Model file for the job. Use its own axes, mm. A direction names the side the tool comes from. Give positions to 0.01 mm unless a question says otherwise; leave off trailing zeros. Order: outer loops, then holes, each group sorted by start corner. A loop starts at its lowest first (then second) coordinate and runs counter-clockwise, first axis right, second up. Notation, with made-up numbers: (-9.75, 21.25) - (39.25, 21.25) arc R29 cw to (39.25, 60.25) - close; hole circle Ø1 at (75, 74.5). An arc over 180 degrees is marked (long way). Use CSV: the item, a comma, the result in double quotes. Start each with the question number.
(1) Band-saw the part on B-B, the plane y = -2. Give the cut face in (x, z) (3 decimals), then the cut area to 3 significant figures.
(2) Drop flat-ended pins along their axis: pin 1 Ø2 at (x, z) = (0.5, 0.5) entering from +Y; pin 2 Ø2 at (y, z) = (-3.5, 2) entering from +X; pin 3 Ø1.2 at (x, z) = (-0.5, -0.5) entering from -Y; pin 4 Ø2.5 at (x, z) = (0, -7.5) entering from -Y. Give the stop position or say it passes through.
(3) Band-saw the part on A-A, the plane z = -7.5. Count the separate pieces of the cut face and the enclosed holes in it, then the cut area to 3 significant figures.
(4) Pull direction X, two halves, no side cores. Call faces 5 (the cylindrical face through (0.07, -5.51, -9)), 6 (the flat face through (1, 6, 2)), 7 (the conical face through (-1.88, 0.24, -5.95)), 8 (the cylindrical face through (0, 3, -6)): +X half, -X half, draft (parallel to the pull), parting line (faces both ways), or undercut.
(5) Probe L1, parallel to Y at x = 0, z = 5 (3 decimals); L2, parallel to X at y = 5.4, z = 0; L3, parallel to X at y = 5.7, z = 0. List the from-to ranges inside material, lowest first.
(6) Tool access for faces 1 (the flat face through (0, 1, 1.7)), 2 (the cylindrical face through (0.186, -0.587, 3.808)), 3 (the flat face through (5, -5, 5)), 4 (the flat face through (0, 5, 0)): list every direction of +Z, -Z, +X, -X, +Y, -Y with a clear straight run to the whole face (end or side of a thin tool).
from build123d import *

# Parameters (mm, degrees)
FLAT_GROVE_EXTRUDE_REACH   = 21.647
WIRE_HOLE_CUT_DEPTH        = 20.052558883
WIRE_HOLE_CUT_DEPTH_BACK   = 20.052558883
SKETCH5_R                  = 1.5
SKETCH6_R                  = 1.425
SET_SCREW_CUT_DEPTH        = 18.698870187
MAGNET_START               = -1
SKETCH8_R                  = 11
SKETCH8_R_2                = 3.05
MAGNET_HOLDER_TRIM_DEPTH   = 1
MAGNET_HOLDER_CHAMFER_SIZE = 1
AXLE_TOLERANCE_CUT_DEPTH   = 8


with BuildPart() as part:
    # Sketch1 → Spool Solid (revolve)
    with BuildSketch(Plane(origin=(0, 0, 0), x_dir=(0, 0, -1), z_dir=(1, 0, 0)), mode=Mode.PRIVATE) as spool_solid_sk:
        Polygon((-2.05, 6), (-11, 6), (-11, 5), (-6, 0), (-6, -5), (-11, -5), (-11, -6), (-2, -6), (-2, 2), (0, 4), (0, 5), (-2.05, 5), align=None)
    revolve(spool_solid_sk.sketch.rotate(Axis((0, 0, 0), (0, 1, 0)), 180), axis=Axis((0, 0, 0), (0, 1, 0)))

    # Flat Grove Extrude: up to this cone (the profile starts inside it)
    flat_grove_extrude_end = Plane(origin=(0, -6, 0), z_dir=(0, -1, 0)).offset(-9.999999) * Cone(1e-06, 42.147, 42.146999, align=(Align.CENTER, Align.CENTER, Align.MIN), mode=Mode.PRIVATE)
    # Sketch2 → Flat Grove Extrude (add, up to the surface)
    with BuildSketch(Plane.XZ.offset(6), mode=Mode.PRIVATE) as flat_grove_extrude_sk1:
        with BuildLine():
            Line((1.322875656, 1.5), (-1.322875656, 1.5))
            ThreePointArc((-1.322875656, 1.5), (0, 2), (1.322875656, 1.5))
        make_face()
    flat_grove_extrude_tool1 = extrude(flat_grove_extrude_sk1.sketch, amount=-FLAT_GROVE_EXTRUDE_REACH, mode=Mode.PRIVATE) & flat_grove_extrude_end
    add(flat_grove_extrude_tool1.solids().sort_by_distance((0, -6, 1.702311))[0])

    # Sketch5 → Wire Hole Cut (cut, two sides: drawn at the far end of the back side and taken through both)
    with BuildSketch(Plane(origin=(0, -5, 0), x_dir=(1, 0, 0), z_dir=(0, 1, 0)).offset(-WIRE_HOLE_CUT_DEPTH_BACK)):
        with Locations(Location((0, 7.5, 0), (0, 0, 270))):
            Circle(SKETCH5_R)
    extrude(amount=WIRE_HOLE_CUT_DEPTH + WIRE_HOLE_CUT_DEPTH_BACK, mode=Mode.SUBTRACT)

    # Sketch6 → Set Screw Cut (cut, through all)
    with BuildSketch(Plane(origin=(0, 0, 1.5), x_dir=(-1, 0, 0), z_dir=(0, 0, -1))):
        with Locations((0, -2)):
            Circle(SKETCH6_R)
    extrude(amount=-SET_SCREW_CUT_DEPTH, mode=Mode.SUBTRACT)

    # Sketch8 → Magnet Holder Trim (cut)
    with BuildSketch(Plane(origin=(0, 6, 0), x_dir=(1, 0, 0), z_dir=(0, 1, 0)).offset(MAGNET_START)):
        with Locations(Location((0, 0, 0), (0, 0, 90))):
            Circle(SKETCH8_R)
        with Locations(Location((0, 0, 0), (0, 0, 270))):
            Circle(SKETCH8_R_2, mode=Mode.SUBTRACT)
    extrude(amount=MAGNET_HOLDER_TRIM_DEPTH, mode=Mode.SUBTRACT)

    # Magnet Holder Chamfer
    magnet_holder_chamfer_edges = [part.edges().sort_by_distance(p)[0] for p in [
        (0, 5, -3.05),
    ]]
    chamfer(magnet_holder_chamfer_edges, length=MAGNET_HOLDER_CHAMFER_SIZE - 0.0001)  # a hair under: the kernel refuses the full size

    # Sketch9 → Axle Tolerance Cut (cut)
    with BuildSketch(Plane.XZ.offset(6)):
        with BuildLine():
            Line((1.396424004, 1.7), (-1.396424004, 1.7))
            ThreePointArc((-1.396424004, 1.7), (0, -2.2), (1.396424004, 1.7))
        make_face()
    extrude(amount=-AXLE_TOLERANCE_CUT_DEPTH, mode=Mode.SUBTRACT)


solid = part.part
Answer block:
1,outline,"(-1.425, 1.676) - (-1.425, 5.828) arc R6 ccw (long way) to (1.425, 5.828) - (1.425, 1.676) arc R2.2 cw (long way) to start"
1,area,"86.8 mm2"
2,pin 1,"stops at y = 5"
2,pin 2,"stops at x = 5.92"
2,pin 3,"stops at y = 2.69"
2,pin 4,"passes through"
3,separate pieces,"4"
3,enclosed holes,"0"
3,area,"38.8 mm2"
4,face 5,"undercut"
4,face 6,"draft"
4,face 7,"parting line"
4,face 8,"undercut"
5,L1,"y = -6 to -3.425, -0.575 to 5"
5,L2,"x = -3.65 to -2.05, 2.05 to 3.65"
5,L3,"x = -3.35 to -2.05, 2.05 to 3.35"
6,face 1,"-Y"
6,face 2,"+Z"
6,face 3,"none"
6,face 4,"+Y"
